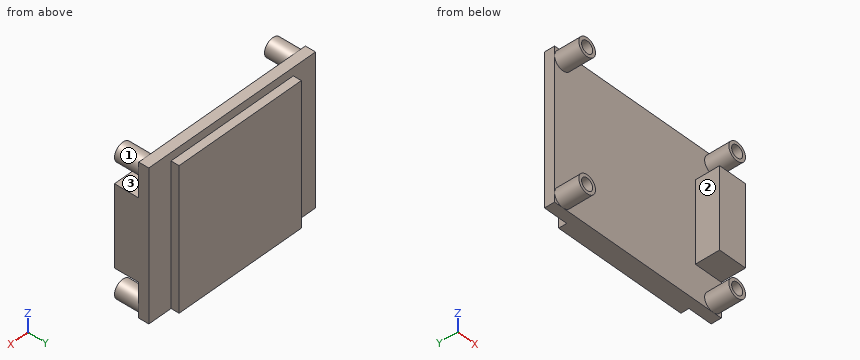
from build123d import *

# Parameters (mm, degrees)
SKETCH_1_W      = 45
SKETCH_1_H      = 37
EXTRUDE_1_DEPTH = 2.5
SKETCH_2_W      = 33
SKETCH_2_H      = 35
EXTRUDE_2_DEPTH = 2
SKETCH_3_R      = 2.25
SKETCH_3_R_2    = 1.5
SKETCH_3_W      = 7
SKETCH_3_H      = 20
EXTRUDE_3_DEPTH = 6


with BuildPart() as part:
    # 草图1 → 凸台-拉伸1 (new body)
    with BuildSketch(Plane(origin=(0, 0, 0), x_dir=(1, 0, 0), z_dir=(0, 1, 0))):
        with Locations((22.5, 18.5)):
            Rectangle(SKETCH_1_W, SKETCH_1_H)
    extrude(amount=EXTRUDE_1_DEPTH)

    # 草图2 → 凸台-拉伸2 (add)
    with BuildSketch(Plane(origin=(0, 2.5, 0), x_dir=(1, 0, 0), z_dir=(0, 1, 0))):
        with Locations((22.5, 19.5)):
            Rectangle(SKETCH_2_W, SKETCH_2_H)
    extrude(amount=EXTRUDE_2_DEPTH)

    # 草图3 → 凸台-拉伸3 (add)
    # profile 1 of 5: a face of its own
    with BuildSketch(Plane.XZ):
        with Locations(Location((42.75, -34.75, 0), (0, 0, 270))):
            Circle(SKETCH_3_R)
        with Locations(Location((42.75, -34.75, 0), (0, 0, 270))):
            Circle(SKETCH_3_R_2, mode=Mode.SUBTRACT)
    # profile 2 of 5: a face of its own
    with BuildSketch(Plane.XZ):
        with Locations(Location((42.75, -2.25, 0), (0, 0, 90))):
            Circle(SKETCH_3_R)
        with Locations(Location((42.75, -2.25, 0), (0, 0, 90))):
            Circle(SKETCH_3_R_2, mode=Mode.SUBTRACT)
    # profile 3 of 5: a face of its own
    with BuildSketch(Plane.XZ):
        with Locations(Location((2.25, -2.25, 0), (0, 0, 90))):
            Circle(SKETCH_3_R)
        with Locations(Location((2.25, -2.25, 0), (0, 0, 270))):
            Circle(SKETCH_3_R_2, mode=Mode.SUBTRACT)
    # profile 4 of 5: a face of its own
    with BuildSketch(Plane.XZ):
        with Locations(Location((2.25, -34.75, 0), (0, 0, 90))):
            Circle(SKETCH_3_R)
        with Locations(Location((2.25, -34.75, 0), (0, 0, 90))):
            Circle(SKETCH_3_R_2, mode=Mode.SUBTRACT)
    # profile 5 of 5: a face of its own
    with BuildSketch(Plane.XZ):
        with Locations((41.5, -18.5)):
            Rectangle(SKETCH_3_W, SKETCH_3_H)
    extrude(amount=EXTRUDE_3_DEPTH)


solid = part.part
Could you check a few things on this model? Use its own coordinates, in mm. Face numbers are marked on the shaded views. A direction names the side the tool comes from. Give positions to 0.01 mm unless a question says otherwise; leave off trailing zeros. Write each loop counter-clockwise with the first axis right and the second up, starting at its lowest first coordinate (ties: lowest second). Pieces come first, ordered by that corner, then holes. Notation, with made-up numbers: (89, -25.5) -> (97, -25.5) arc R20 cw to (97, 2.5) -> close; hole circle Ø3 at (2.25, -11). An arc over 180 degrees is marked (long way). Answer as a JSON object with one key per item and string values.
Q1. Which directions (+Z, -Z, +X, -X, +Y, -Y) give clear straight access to the entire face, cutting with the end or side of a thin tool? Please do the marked faces 1, 2 and 3.
Taken from the geometry:
{"face 1": "-Y", "face 2": "+Z, -Z, -X, -Y", "face 3": "+X, -X, -Y"}
Q2. Please list where these lines run through material, in increasing order: L1, parallel to X at y = -3.05, z = -2.25; L2, parallel to Y at x = 9, z = -21; L3, parallel to Y at x = 4.5, z = -14.5.
Taken from the geometry:
{"L1": "x = 0 to 0.75, 3.75 to 4.5, 40.5 to 41.25, 44.25 to 45", "L2": "y = 0 to 4.5", "L3": "y = 0 to 2.5"}
Q3. Suppose I cut it at C-C on x = 33.5. Write out the boundary of the cut face in (y, z), then the cut area to 4 significant figures.
Taken from the geometry:
{"outline": "(0, -37) -> (4.5, -37) -> (4.5, -2) -> (2.5, -2) -> (2.5, 0) -> (0, 0) -> close", "area": "162.5 mm²"}
Q4. Suppose I cut it at A-A on y = -4.25. Count the separate pieces of the cut face and the enclosed holes in it, then the cut area to 3 significant figures.
Taken from the geometry:
{"separate pieces": "5", "enclosed holes": "4", "area": "175 mm²"}
Q5. Suppose I cut it at B-B on z = -30. Write out the boundary of the cut face in (x, y), then the cut area to 4 significant figures.
Taken from the geometry:
{"outline": "(0, 0) -> (45, 0) -> (45, 2.5) -> (39, 2.5) -> (39, 4.5) -> (6, 4.5) -> (6, 2.5) -> (0, 2.5) -> close", "area": "178.5 mm²"}
Q6. Will these pins go through, and if not, where does the flat tip stop? pin 1 Ø8 at (x, z) = (19, -30) entering from -Y; pin 2 Ø1.6 at (y, z) = (3.5, -23.5) entering from +X; pin 3 Ø6 at (x, y) = (17.5, -2) entering from +Z; pin 4 Ø1.8 at (x, y) = (41, -3.5) entering from -Z.
Taken from the geometry:
{"pin 1": "stops at y = 0", "pin 2": "stops at x = 39", "pin 3": "stops at z = 0", "pin 4": "stops at z = -36.83"}
